Geometry check sheet. Reference: the model listing, model coordinates, mm. Face numbers are marked on the shaded views. A direction names the side the tool comes from. Round coordinates to 2 decimals unless told otherwise and drop trailing zeros. Order: outer loops, then holes, each group sorted by start corner. A loop starts at its lowest first (then second) coordinate and runs counter-clockwise, first axis right, second up. Notation, with made-up numbers: (17, 34) -> (64, 34) arc R15 cw to (64, 55) -> close; hole circle Ø6 at (-37.75, -34.75). An arc over 180 degrees is marked (long way). Answer as a JSON object with one key per item and string values. Group by question number.
from build123d import *

# Parameters (mm, degrees)
F1_DEPTH = 2
F3_DEPTH = 12
F4_R     = 3.5
F5_DEPTH = 10
F6_R     = 2.5
F7_DEPTH = 18.001


with BuildPart() as f1:
    # F0 (on Top) → F1 (new body)
    with BuildSketch(Plane.XY):
        Polygon((0, 18), (0, 0), (18, 0), align=None)
    extrude(amount=F1_DEPTH)

    # F2 (on face) → F3 (join)
    with BuildSketch(Plane.XY.offset(2)):
        Polygon((0, 18), (0, 0), (18, 0), (15, 3), (3, 3), (3, 15), align=None)
    extrude(amount=F3_DEPTH)

    # F4 (on face) → F5 (join)
    with BuildSketch(Plane(origin=(0, 0, 0), x_dir=(0, -1, 0), z_dir=(-1, 0, 0))):
        with Locations((-12, 7)):
            Circle(F4_R)
    extrude(amount=F5_DEPTH)

    # F6 (on face) → F7 (cut, through all)
    with BuildSketch(Plane.XZ):
        with Locations((12, 6.5)):
            Circle(F6_R)
    extrude(amount=-F7_DEPTH, mode=Mode.SUBTRACT)


solid = f1.part
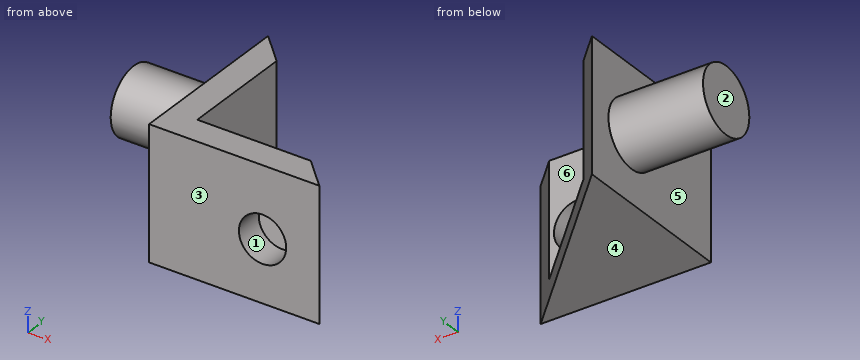
Item 1: Sectioned sample at D-D, the plane x = 6.25. Enter the section's corners in (y, z).
Item 2: Sectioned sample at A-A, the plane x = 12. Enter the section's corners in (y, z), then the cut area to 3 significant figures.
Item 3: Sectioned sample at C-C, the plane y = 4.75. Enter the section's corners in (x, z).
Item 4: Mould release check, pull along X, two halves, no side actions. Record for the marked faces 1, 2 and 3: pulls with the +X half, pulls with the -X half, needs draft (parallel to the pull), parting line crosses it, or undercut.
Item 5: Thickness scan on L1, parallel to Z at x = 12, y = 2.1; L2, parallel to Y at x = 2.5, z = 3.5; L3, parallel to X at y = 11.25, z = 12. Record the ranges inside material, lowest first.
Item 6: Depth check by flat-ended pin: pin 1 Ø8 at (x, z) = (12, 6.5) entering from +Y; pin 2 Ø5 at (y, z) = (7.5, 10) entering from +X; pin 3 Ø2 at (y, z) = (10.5, 2.5) entering from +X. Enter the tip coordinate at first touch or a pass-through.
Item 7: Set-up check for the marked faces 4, 5 and 6: record each of +Z, -Z, +X, -X, +Y, -Y from which the full face is reachable in a straight line by a thin tool's end or side.
Item 8: Sectioned sample at B-B, the plane z = 6.5. Enter the section's corners in (x, y).
Result:
{
 "1": {"outline": "(0, 0) -> (11.75, 0) -> (11.75, 2) -> (3, 2) -> (3, 14) -> (0, 14) -> close"},
 "2": {"outline": "(0, 0) -> (6, 0) -> (6, 2) -> (3, 2) -> (3, 4) -> (0, 4) -> close; (0, 9) -> (3, 9) -> (3, 14) -> (0, 14) -> close", "area": "33.0 mm2"},
 "3": {"outline": "(0, 0) -> (13.25, 0) -> (13.25, 2) -> (3, 2) -> (3, 14) -> (0, 14) -> close"},
 "4": {"face 1": "undercut", "face 2": "pulls with the -X half", "face 3": "needs draft"},
 "5": {"L1": "z = 0 to 4, 9 to 14", "L2": "y = 0 to 15.5", "L3": "x = 0 to 3"},
 "6": {"pin 1": "stops at y = 3", "pin 2": "stops at x = 3", "pin 3": "stops at x = 8.37"},
 "7": {"face 4": "-Z, +X, -X, +Y, -Y", "face 5": "-X", "face 6": "+Z, +X, +Y"},
 "8": {"outline": "(-10, 8.54) -> (0, 8.54) -> (0, 0) -> (9.5, 0) -> (9.5, 3) -> (3, 3) -> (3, 15) -> (0, 18) -> (0, 15.46) -> (-10, 15.46) -> close; (14.5, 0) -> (18, 0) -> (15, 3) -> (14.5, 3) -> close"}
}
